Build history of the part. All positions in model axes, mm. Coordinates: 2 decimals unless noted, no trailing zeros. Order: outer loops, then holes, each group sorted by start corner. A loop starts at its lowest first (then second) coordinate and runs counter-clockwise, first axis right, second up. Notation, with made-up numbers: (-25.5, 72) - (-12.5, 72) arc R24 ccw to (-12.5, 100) - close; hole circle Ø1 at (-15, 32). An arc over 180 degrees is marked (long way). One line per item, written item: value.
from build123d import *

# Parameters (mm, degrees)
SKETCH1_R           = 90
BOSS_EXTRUDE1_DEPTH = 3
SKETCH2_W           = 3
SKETCH2_H           = 14
CUT_EXTRUDE2_DEPTH  = 3
CIRPATTERN1_COUNT   = 8
SKETCH16_W          = 3
SKETCH16_H          = 5
CUT_EXTRUDE5_DEPTH  = 3
CIRPATTERN2_COUNT   = 8
SKETCH24_R          = 50
CUT_EXTRUDE6_DEPTH  = 3


with BuildPart() as part:
    # Sketch1 → Boss-Extrude1 (new body)
    with BuildSketch(Plane(origin=(0, 0, 0), x_dir=(1, 0, 0), z_dir=(0, 1, 0))):
        Circle(SKETCH1_R)
    extrude(amount=BOSS_EXTRUDE1_DEPTH)

    # Sketch2 → Cut-Extrude2 (cut)
    with BuildSketch(Plane(origin=(0, 3, 0), x_dir=(1, 0, 0), z_dir=(0, 1, 0))):
        with Locations((0, 70)):
            Rectangle(SKETCH2_W, SKETCH2_H)
    cut_extrude2 = extrude(amount=-CUT_EXTRUDE2_DEPTH, mode=Mode.SUBTRACT)

    # CirPattern1: Cut-Extrude2 ×8 about axis
    cirpattern1_axis = Axis((0, 0, 0), (0, 1, 0))
    for i in range(1, CIRPATTERN1_COUNT):
        add(cut_extrude2.rotate(cirpattern1_axis, i * 360 / CIRPATTERN1_COUNT), mode=Mode.SUBTRACT)

    # Sketch16 → Cut-Extrude5 (cut)
    with BuildSketch(Plane(origin=(0, 3, 0), x_dir=(1, 0, 0), z_dir=(0, 1, 0))):
        with Locations((-4, 82.5)):
            Rectangle(SKETCH16_W, SKETCH16_H)
        with Locations((4, 82.5)):
            Rectangle(SKETCH16_W, SKETCH16_H)
        with Locations((-4, 57.5)):
            Rectangle(SKETCH16_W, SKETCH16_H)
        with Locations((4, 57.5)):
            Rectangle(SKETCH16_W, SKETCH16_H)
    cut_extrude5 = extrude(amount=-CUT_EXTRUDE5_DEPTH, mode=Mode.SUBTRACT)

    # CirPattern2: Cut-Extrude5 ×8 about axis
    cirpattern2_axis = Axis((0, 0, 0), (0, 1, 0))
    for i in range(1, CIRPATTERN2_COUNT):
        add(cut_extrude5.rotate(cirpattern2_axis, i * 360 / CIRPATTERN2_COUNT), mode=Mode.SUBTRACT)

    # Sketch24 → Cut-Extrude6 (cut)
    with BuildSketch(Plane(origin=(0, 3, 0), x_dir=(1, 0, 0), z_dir=(0, 1, 0))):
        Circle(SKETCH24_R)
    extrude(amount=-CUT_EXTRUDE6_DEPTH, mode=Mode.SUBTRACT)


solid = part.part
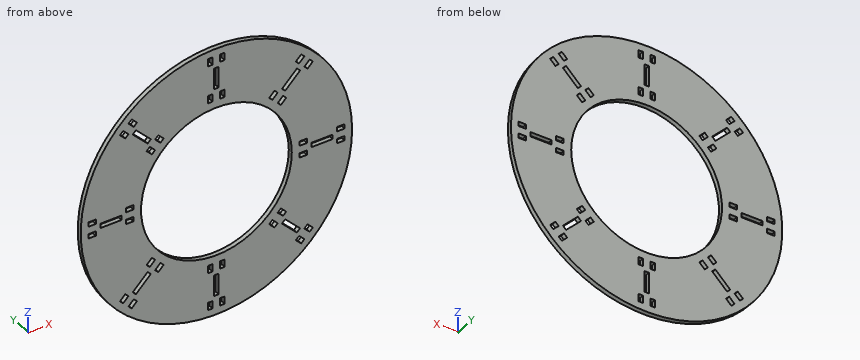
1. Band-saw the part on B-B, the plane z = -17. Give the cut face in (x, y).
Values found:
outline: (-88.38, 0) - (-47.02, 0) - (-47.02, 3) - (-88.38, 3) - close; (47.02, 0) - (88.38, 0) - (88.38, 3) - (47.02, 3) - close
2. Probe line 1 along Z through (x, y) = (0, 1.9); line 2 along Z through (x, y) = (-42.5, 1.75). List the from-to ranges inside material, lowest first.
Values found:
line 1: z = -90 to -77, -63 to -50, 50 to 63, 77 to 90
line 2: z = -79.33 to -38.96, -35.28 to -26.34, 26.34 to 35.28, 38.96 to 79.33
3. Band-saw the part on C-C, the plane y = 1.85. Count the separate pieces of the cut face and the enclosed holes in it, and give its area (3 significant figures).
Values found:
separate pieces: 1
enclosed holes: 41
area: 16,800 mm2
4. Band-saw the part on A-A, the plane x = -74.5. Give the cut face in (y, z).
Values found:
outline: (0, -50.5) - (3, -50.5) - (3, -1.5) - (0, -1.5) - close; (0, 1.5) - (3, 1.5) - (3, 50.5) - (0, 50.5) - close
5. Flat gauge pins, fed straight in: P1, Ø10, axis at x = -5, z = -59, coming from the -Y side; P2, Ø1.5, axis at x = 4, y = 1.5, coming from the +Z side; P3, Ø0.9, axis at y = 2, z = 4, coming from the -X side; P4, Ø1.5, axis at x = -82.5, y = 1, coming from the -Z side. Where does each tip first touch, or does it go through?
Values found:
P1: stops at y = 0
P2: stops at z = 89.94
P3: stops at x = -89.93
P4: stops at z = -37.64
